Could you check a few things on this model? Use its own coordinates, in mm. Face numbers are marked on the shaded views. A direction names the side the tool comes from. Round coordinates to 2 decimals unless told otherwise and drop trailing zeros. Write each loop counter-clockwise with the first axis right and the second up, starting at its lowest first coordinate (ties: lowest second). Pieces come first, ordered by that corner, then holes. Notation, with made-up numbers: (24.25, -4.75) -> (80.25, -4.75) arc R10 cw to (80.25, 3.25) -> close; hole circle Ø7 at (23.25, 65.5). An arc over 180 degrees is marked (long way). Return JSON: item names as keys, results as strings.
from build123d import *

# Parameters (mm, degrees)
F0_W        = 25.4
F0_H        = 25.4
F1_DEPTH    = 38.1
F0_R        = 5.8024107256
F2_DEPTH    = 127
F3_DEPTH    = 127
F5_DEPTH    = 0.635
F7_DEPTH    = 0.635
F8_F1_R     = 5.08
F8_F2_R     = 5.08
F9_T1_DEPTH = 29.2466340732
F9_T3_DEPTH = 49.2393659268
F9_T5_DEPTH = 11.684
F9_T7_DEPTH = 11.684
F11_DEPTH   = 25.4
F13_DEPTH   = 25.4


# Not quite as in the source:
# - a fillet or chamfer that OpenCascade refuses, or shapes differently, is made with other operations: its cross-section is extruded or revolved along the edge and cut away or added


with BuildPart() as f1:
    # F0 (on Front) → F1 (new body)
    with BuildSketch(Plane.XZ):
        Rectangle(F0_W, F0_H)
        Polygon((7.9375, 7.9375), (7.9375, 0), (7.9375, -7.9375), (0, -7.9375), (-7.9375, -7.9375), (-7.9375, 0), (-7.9375, 7.9375), (0, 7.9375), align=None, mode=Mode.SUBTRACT)
    extrude(amount=F1_DEPTH)



with BuildPart() as f1b:
    # F0 (on Front) → F1, piece 2 (new body)
    with BuildSketch(Plane.XZ):
        with BuildLine():
            ThreePointArc((0, -7.9375), (5.6126600757, -5.6126600757), (7.9375, 0))
            ThreePointArc((7.9375, 0), (5.6126600757, 5.6126600757), (0, 7.9375))
            ThreePointArc((0, 7.9375), (-5.6126600757, 5.6126600757), (-7.9375, 0))
            ThreePointArc((-7.9375, 0), (-5.6126600757, -5.6126600757), (0, -7.9375))
        make_face()
        Circle(F0_R, mode=Mode.SUBTRACT)
    extrude(amount=F1_DEPTH)


with BuildPart() as f1_1:
    add(f1.part)

    add(f1b.part)  # F2 merges F1b
    # F0 (on Front) → F2 (join)
    with BuildSketch(Plane.XZ):
        with BuildLine():
            ThreePointArc((0, -7.9375), (5.6126600757, -5.6126600757), (7.9375, 0))
            ThreePointArc((7.9375, 0), (5.6126600757, 5.6126600757), (0, 7.9375))
            ThreePointArc((0, 7.9375), (-5.6126600757, 5.6126600757), (-7.9375, 0))
            ThreePointArc((-7.9375, 0), (-5.6126600757, -5.6126600757), (0, -7.9375))
        make_face()
        Circle(F0_R, mode=Mode.SUBTRACT)
    extrude(amount=F2_DEPTH)

    # F0 (on Front) → F3 (join)
    with BuildSketch(Plane.XZ):
        with BuildLine():
            Line((7.9375, -7.9375), (7.9375, 0))
            ThreePointArc((7.9375, 0), (5.6126600757, -5.6126600757), (0, -7.9375))
            Line((0, -7.9375), (7.9375, -7.9375))
        make_face()
        with BuildLine():
            ThreePointArc((0, 7.9375), (5.6126600757, 5.6126600757), (7.9375, 0))
            Line((7.9375, 0), (7.9375, 7.9375))
            Line((7.9375, 7.9375), (0, 7.9375))
        make_face()
        with BuildLine():
            ThreePointArc((-7.9375, 0), (-5.6126600757, 5.6126600757), (0, 7.9375))
            Line((0, 7.9375), (-7.9375, 7.9375))
            Line((-7.9375, 7.9375), (-7.9375, 0))
        make_face()
        with BuildLine():
            Line((-7.9375, -7.9375), (0, -7.9375))
            ThreePointArc((0, -7.9375), (-5.6126600757, -5.6126600757), (-7.9375, 0))
            Line((-7.9375, 0), (-7.9375, -7.9375))
        make_face()
    extrude(amount=F3_DEPTH)

    # F4 (on face) → F5 (cut)
    with BuildSketch(Plane(origin=(-7.9375, 0, 0), x_dir=(0, -1, 0), z_dir=(-1, 0, 0))):
        Polygon((106.8973659268, -7.9375), (114.3, 7.9375), (107.95, 7.9375), (100.5473659268, -7.9375), align=None)
        Polygon((98.0073659268, -7.9375002533), (105.41, 7.9374997467), (99.06, 7.9374997467), (91.6573659268, -7.9375002533), align=None)
        Polygon((89.1173659268, -7.9375002533), (96.52, 7.9374997467), (90.17, 7.9374997467), (82.7673659268, -7.9375002533), align=None)
    extrude(amount=-F5_DEPTH, mode=Mode.SUBTRACT)

    # F6 (on face) → F7 (cut)
    with BuildSketch(Plane.YZ.offset(7.9375)):
        Polygon((-107.95, 7.9375), (-114.3, 7.9375), (-106.8973659268, -7.9375), (-100.5473659268, -7.9375), align=None)
        Polygon((-99.06, 7.9374997467), (-105.41, 7.9374997467), (-98.0073659268, -7.9375002533), (-91.6573659268, -7.9375002533), align=None)
        Polygon((-90.17, 7.9374997467), (-96.52, 7.9374997467), (-89.1173659268, -7.9375002533), (-82.7673659268, -7.9375002533), align=None)
    extrude(amount=-F7_DEPTH, mode=Mode.SUBTRACT)

    # F8: fillet of radius 5.08 on 8 edges, made by hand

    # F8_f1
    f8_f1_edges = [f1_1.edges().sort_by_distance(p)[0] for p in [
        (-7.9375, -120.65, 7.9375),
    ]]
    fillet(f8_f1_edges, radius=F8_F1_R)

    # F8_f2
    f8_f2_edges = [f1_1.edges().sort_by_distance(p)[0] for p in [
        (7.9375, -120.65, 7.9375),
    ]]
    fillet(f8_f2_edges, radius=F8_F2_R)

    # F9: fillet of radius 0.762 on 8 edges, made by hand

    # F9_s2 → F9_t1 (cut)
    with BuildSketch(Plane.XZ.offset(102.3253659268)):
        with BuildLine():
            ThreePointArc((-7.9375, -7.1755), (-7.7143153673, -7.7143153673), (-7.1755, -7.9375))
            Line((-7.1755, -7.9375), (-7.1755, -7.95274))
            Line((-7.1755, -7.95274), (-7.95274, -7.95274))
            Line((-7.95274, -7.95274), (-7.95274, -7.1755))
            Line((-7.95274, -7.1755), (-7.9375, -7.1755))
        make_face()
        with BuildLine():
            ThreePointArc((7.9375, -7.1755), (7.7143153673, -7.7143153673), (7.1755, -7.9375))
            Line((7.1755, -7.9375), (7.1755, -7.95274))
            Line((7.1755, -7.95274), (7.95274, -7.95274))
            Line((7.95274, -7.95274), (7.95274, -7.1755))
            Line((7.95274, -7.1755), (7.9375, -7.1755))
        make_face()
    extrude(amount=F9_T1_DEPTH, mode=Mode.SUBTRACT)

    # F9_s4 → F9_t3 (cut)
    with BuildSketch(Plane.XZ.offset(38.1)):
        with BuildLine():
            ThreePointArc((7.1755, -7.9375), (7.7143153673, -7.7143153673), (7.9375, -7.1755))
            Line((7.9375, -7.1755), (7.95274, -7.1755))
            Line((7.95274, -7.1755), (7.95274, -7.95274))
            Line((7.95274, -7.95274), (7.1755, -7.95274))
            Line((7.1755, -7.95274), (7.1755, -7.9375))
        make_face()
        with BuildLine():
            ThreePointArc((-7.1755, -7.9375), (-7.7143153673, -7.7143153673), (-7.9375, -7.1755))
            Line((-7.9375, -7.1755), (-7.95274, -7.1755))
            Line((-7.95274, -7.1755), (-7.95274, -7.95274))
            Line((-7.95274, -7.95274), (-7.1755, -7.95274))
            Line((-7.1755, -7.95274), (-7.1755, -7.9375))
        make_face()
    extrude(amount=F9_T3_DEPTH, mode=Mode.SUBTRACT)

    # F9_s6 → F9_t5 (cut)
    with BuildSketch(Plane.XZ.offset(84.5453659268)):
        with BuildLine():
            ThreePointArc((7.1755, -7.9375), (7.7143153673, -7.7143153673), (7.9375, -7.1755))
            Line((7.9375, -7.1755), (7.95274, -7.1755))
            Line((7.95274, -7.1755), (7.95274, -7.95274))
            Line((7.95274, -7.95274), (7.1755, -7.95274))
            Line((7.1755, -7.95274), (7.1755, -7.9375))
        make_face()
        with BuildLine():
            ThreePointArc((-7.1755, -7.9375), (-7.7143153673, -7.7143153673), (-7.9375, -7.1755))
            Line((-7.9375, -7.1755), (-7.95274, -7.1755))
            Line((-7.95274, -7.1755), (-7.95274, -7.95274))
            Line((-7.95274, -7.95274), (-7.1755, -7.95274))
            Line((-7.1755, -7.95274), (-7.1755, -7.9375))
        make_face()
    extrude(amount=F9_T5_DEPTH, mode=Mode.SUBTRACT)

    # F9_s8 → F9_t7 (cut)
    with BuildSketch(Plane.XZ.offset(93.4353659268)):
        with BuildLine():
            ThreePointArc((7.1755, -7.9375), (7.7143153673, -7.7143153673), (7.9375, -7.1755))
            Line((7.9375, -7.1755), (7.95274, -7.1755))
            Line((7.95274, -7.1755), (7.95274, -7.95274))
            Line((7.95274, -7.95274), (7.1755, -7.95274))
            Line((7.1755, -7.95274), (7.1755, -7.9375))
        make_face()
        with BuildLine():
            ThreePointArc((-7.1755, -7.9375), (-7.7143153673, -7.7143153673), (-7.9375, -7.1755))
            Line((-7.9375, -7.1755), (-7.95274, -7.1755))
            Line((-7.95274, -7.1755), (-7.95274, -7.95274))
            Line((-7.95274, -7.95274), (-7.1755, -7.95274))
            Line((-7.1755, -7.95274), (-7.1755, -7.9375))
        make_face()
    extrude(amount=F9_T7_DEPTH, mode=Mode.SUBTRACT)

    # F10 (on face) → F11 (cut)
    with BuildSketch(Plane(origin=(-7.9375, 0, 0), x_dir=(0, -1, 0), z_dir=(-1, 0, 0))):
        Polygon((139.3916606903, 2.8575), (129.1201191025, 15.1211110401), (129.6502673187, -9.5306912246), align=None)
    extrude(amount=-F11_DEPTH, mode=Mode.SUBTRACT)

    # F12 (on face) → F13 (cut)
    with BuildSketch(Plane(origin=(-7.9375, 0, 0), x_dir=(0, -1, 0), z_dir=(-1, 0, 0))):
        Polygon((131.4901411533, -9.1816671193), (131.4901411533, 8.4584709257), (123.7966120243, 0), (123.7966120243, -4.5106001198), (121.0489347577, -12.0942108333), align=None)
    extrude(amount=-F13_DEPTH, mode=Mode.SUBTRACT)


solid = f1_1.part
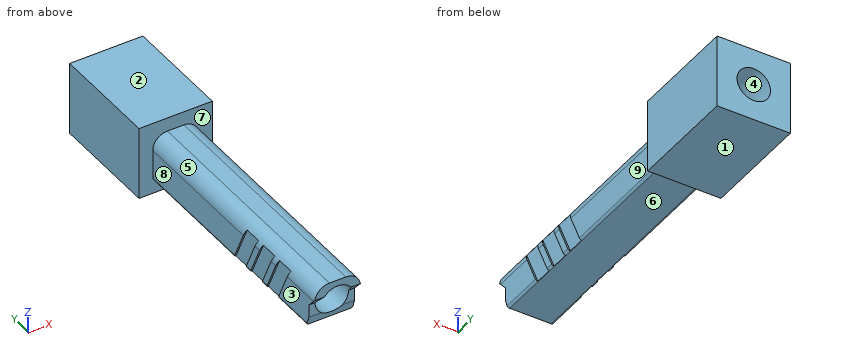
1) For the marked faces 5, 6, 7, 8 and 9, which set-ups out of +Z, -Z, +X, -X, +Y, -Y let a thin tool reach every point of the face, with its end or its side?
Return value:
{"face 5": "+Z, -X, -Y", "face 6": "-Z, +X, -X, -Y", "face 7": "-Y", "face 8": "+Z, -Z, -X, -Y", "face 9": "+Z, -Z, +X, -Y"}
2) Will these pins go through, and if not, where does the flat tip stop? pin 1 Ø14 at (y, z) = (-99.5, -2) entering from +X; pin 2 Ø4 at (y, z) = (-65, 5.5) entering from -X; pin 3 Ø3 at (x, y) = (-0.5, -91) entering from +Z.
Return value:
{"pin 1": "x = 7.94", "pin 2": "x = -7.9", "pin 3": "z = 7.94"}
3) I want a section at D-D, the plane z = 9.25. Please give me the cut outline in (x, y).
Return value:
{"outline": "(-12.7, -38.1) -> (12.7, -38.1) -> (12.7, 0) -> (-12.7, 0) -> close"}
4) I want a section at A-A, the plane y = -16. Please give me the cut outline in (x, z), and give its area (3 significant figures).
Return value:
{"outline": "(-12.7, -12.7) -> (12.7, -12.7) -> (12.7, 12.7) -> (-12.7, 12.7) -> close; hole circle Ø11.6 at (0, 0)", "area": "539 mm²"}
5) I want a section at B-B, the plane x = 0. Please give me the cut outline in (y, z).
Return value:
{"outline": "(-127, 5.8) -> (0, 5.8) -> (0, 12.7) -> (-38.1, 12.7) -> (-38.1, 7.94) -> (-127, 7.94) -> close; (-123.33, -5.8) -> (-122.55, -7.94) -> (-38.1, -7.94) -> (-38.1, -12.7) -> (0, -12.7) -> (0, -5.8) -> close"}
6) If I drill on probe 1 along X at (y, z) = (-48.5, 0); probe 2 along Y at (x, z) = (2, -11.25), over which ranges is the centre line in solid material (lowest first)? Write a range as [from, to].
Return value:
{"probe 1": "[-7.94, -5.8], [5.8, 7.94]", "probe 2": "[-38.1, 0]"}
7) Thinking about a two-plate mould opening in Z: for the marked faces 1, 2, 3 and 4, which applies, pulls with the +Z half, pulls with the -Z half, needs draft (parallel to the pull), parting line crosses it, or undercut?
Return value:
{"face 1": "pulls with the -Z half", "face 2": "pulls with the +Z half", "face 3": "needs draft", "face 4": "undercut"}
8) I want a section at C-C, the plane y = -41. Please give me the cut outline in (x, z), and give its area (3 significant figures).
Return value:
{"outline": "(-7.94, -7.18) arc R0.76 ccw to (-7.18, -7.94) -> (7.18, -7.94) arc R0.76 ccw to (7.94, -7.18) -> (7.94, 2.86) arc R5.08 ccw to (2.86, 7.94) -> (-2.86, 7.94) arc R5.08 ccw to (-7.94, 2.86) -> close; hole circle Ø11.6 at (0, 0)", "area": "135 mm²"}
